```python
from build123d import *

# Parameters (mm, degrees)
BOSS_EXTRUDE1_DEPTH = 3
SKETCH2_R           = 8
SKETCH2_R_2         = 1
CUT_EXTRUDE1_DEPTH  = 3


with BuildPart() as part:
    # Sketch1 → Boss-Extrude1 (new body)
    with BuildSketch(Plane(origin=(0, 0, 0), x_dir=(1, 0, 0), z_dir=(0, 1, 0))):
        Polygon((-41, -41), (-17.5, -41), (-17.5, -38), (17.5, -38), (17.5, -41), (41, -41), (41, -17.5), (38, -17.5), (38, 17.5), (41, 17.5), (41, 41), (17.5, 41), (17.5, 38), (-17.5, 38), (-17.5, 41), (-41, 41), (-41, 17.5), (-38, 17.5), (-38, -17.5), (-41, -17.5), align=None)
    extrude(amount=BOSS_EXTRUDE1_DEPTH)

    # Sketch2 → Cut-Extrude1 (cut)
    with BuildSketch(Plane(origin=(0, 3, 0), x_dir=(1, 0, 0), z_dir=(0, 1, 0))):
        with Locations((-13, 0)):
            Circle(SKETCH2_R)
        with Locations((-21, 8.5)):
            Circle(SKETCH2_R_2)
        with Locations((-21, -8.5)):
            Circle(SKETCH2_R_2)
        with Locations((21, -8.5)):
            Circle(SKETCH2_R_2)
        with Locations((21, 8.5)):
            Circle(SKETCH2_R_2)
        with Locations((13, 0)):
            Circle(SKETCH2_R)
    extrude(amount=-CUT_EXTRUDE1_DEPTH, mode=Mode.SUBTRACT)


solid = part.part
```
Could you check a few things on this model? Use its own coordinates, in mm. A direction names the side the tool comes from. Round coordinates to 2 decimals unless told otherwise and drop trailing zeros. Loops run counter-clockwise (first coordinate to the right, second up) from the corner with the lowest first, then second, coordinate; pieces in that order, holes last.
Q1. I want a section at B-B (y = 2.35). Write out the boundary of the cut face in (x, z).
Q2. I want a section at C-C (z = 0). Write out the boundary of the cut face in (x, y).
Q3. I want a section at A-A (x = -13). Write out the boundary of the cut face in (y, z), and give its area (3 significant figures).
Q4. On a 3-axis mill with a long thin cutter (end or side, diameter ignored), from which of +Z, -Z, +X, -X, +Y, -Y can I reach the whole of each face in a straight line? I mean faces 5 (the flat face through (40, 1, 17.5)), 6 (the flat face through (0, 1, 38)), 7 (the flat face through (-17.5, 1, -39)). Say none if no direction works.
Q5. Please list where these lines run through material, in increasing order: L1, parallel to X at y = 1.05, z = 0; L2, parallel to X at y = 1, z = 8.5; L3, parallel to X at y = 2.85, z = 38.5.
Q6. I want a section at D-D (z = 16). Write out the boundary of the cut face in (x, y), and give its area (3 significant figures).
Q7. For P1, Ø1.5, axis at x = 11, y = 2.5, coming from the -Z side; P2, Ø1.5, axis at y = 1, z = -14, coming from the -X side, each with a flat end and sliding along its axis, tell me the tip position at first contact or that it passes through.
Q8. Thinking about a two-plate mould opening in X: for faces 1 (the flat face through (-41, 1, -29)), 2 (the flat face through (41, 1, -29)), 3 (the cylindrical face through (-21.13, 1.52, -9.49)), 4 (the flat face through (29, 1, -41)), which applies, pulls with the +X half, pulls with the -X half, needs draft (parallel to the pull), parting line crosses it, or undercut?
Answer below:
1. outline: (-41, -41) - (-17.5, -41) - (-17.5, -38) - (17.5, -38) - (17.5, -41) - (41, -41) - (41, -17.5) - (38, -17.5) - (38, 17.5) - (41, 17.5) - (41, 41) - (17.5, 41) - (17.5, 38) - (-17.5, 38) - (-17.5, 41) - (-41, 41) - (-41, 17.5) - (-38, 17.5) - (-38, -17.5) - (-41, -17.5) - close; hole circle Ø2 at (-21, -8.5); hole circle Ø2 at (-21, 8.5); hole circle Ø16 at (-13, 0); hole circle Ø16 at (13, 0); hole circle Ø2 at (21, -8.5); hole circle Ø2 at (21, 8.5)
2. outline: (-38, 0) - (-21, 0) - (-21, 3) - (-38, 3) - close; (-5, 0) - (5, 0) - (5, 3) - (-5, 3) - close; (21, 0) - (38, 0) - (38, 3) - (21, 3) - close
3. outline: (0, -38) - (3, -38) - (3, -8) - (0, -8) - close; (0, 8) - (3, 8) - (3, 38) - (0, 38) - close
3. area: 180 mm2
4. face 5: +X, +Y, -Y
4. face 6: +Z, +Y, -Y
4. face 7: -Z, +Y, -Y
5. L1: x = -38 to -21, -5 to 5, 21 to 38
5. L2: x = -38 to -22, -20 to 20, 22 to 38
5. L3: x = -41 to -17.5, 17.5 to 41
6. outline: (-38, 0) - (38, 0) - (38, 3) - (-38, 3) - close
6. area: 228 mm2
7. P1: stops at z = -38
7. P2: stops at x = -38
8. face 1: pulls with the -X half
8. face 2: pulls with the +X half
8. face 3: undercut
8. face 4: needs draft
